```python
from build123d import *

# Parameters (mm, degrees)
F0_W     = 180
F0_H     = 270
F0_W_2   = 140
F0_H_2   = 230
F1_DEPTH = 11


with BuildPart() as f1:
    # F0 (on Right) → F1 (new body)
    with BuildSketch(Plane.YZ):
        with Locations((-34.164113, -2.262233)):
            Rectangle(F0_W, F0_H)
        with Locations((-34.164113, -2.262233)):
            Rectangle(F0_W_2, F0_H_2, mode=Mode.SUBTRACT)
    extrude(amount=F1_DEPTH)


solid = f1.part
```
Read the model definition and answer for the solid it produces. Units are mm, in the model's axes. A direction names the side the tool comes from. Give positions to 0.01 mm unless a question says otherwise; leave off trailing zeros. Order: outer loops, then holes, each group sorted by start corner. A loop starts at its lowest first (then second) coordinate and runs counter-clockwise, first axis right, second up.
(1) For a pull along Y with two mould halves and no side action, classify faces 3 (the flat face through (5, -124.164, -4)), 4 (the flat face through (5, -35, 132.738)), 5 (the flat face through (5, 35.836, -4)), 6 (the flat face through (5, 55.836, -4)) as released by +Y, released by -Y, zero draft, split by the parting line, or undercut.
(2) Find section C-C (x = 7.75). Give the vertices of the cut face in (y, z), plus the area to 3 significant figures.
(3) Find section B-B (z = -9). Give the vertices of the cut face in (x, y), plus the area to 3 significant figures.
(4) Find section A-A (y = 22). Give the vertices of the cut face in (x, z).
(5) Given pin 1 (10 mm diameter, centred on y = 26, z = 60, fed in from -X), flat-ended and moving along its own axis, determine where the tip first touches the part or whether it passes through.
(6) Straight lines are drawn through the part: L1, parallel to Z at x = 3.25, y = 35.5; L2, parallel to Y at x = 9.75, z = -43. For each, find the intervals that lie inside material, in ascending order.
(7) For faces 1 (the flat face through (5, -35, 112.738)), 2 (the flat face through (11, -115, 0)), determine the directions among +Z, -Z, +X, -X, +Y, -Y from which every point of the face is accessible in a straight line to the end or side of a thin tool.
Result sheet:
1. face 3: released by -Y
1. face 4: zero draft
1. face 5: undercut
1. face 6: released by +Y
2. outline: (-124.16, -137.26) - (55.84, -137.26) - (55.84, 132.74) - (-124.16, 132.74) - close; hole (-104.16, -117.26) - (35.84, -117.26) - (35.84, 112.74) - (-104.16, 112.74) - close
2. area: 16,400 mm2
3. outline: (0, -124.16) - (11, -124.16) - (11, -104.16) - (0, -104.16) - close; (0, 35.84) - (11, 35.84) - (11, 55.84) - (0, 55.84) - close
3. area: 440 mm2
4. outline: (0, -137.26) - (11, -137.26) - (11, -117.26) - (0, -117.26) - close; (0, 112.74) - (11, 112.74) - (11, 132.74) - (0, 132.74) - close
5. pin 1: passes through
6. L1: z = -137.26 to -117.26, 112.74 to 132.74
6. L2: y = -124.16 to -104.16, 35.84 to 55.84
7. face 1: +X, -X
7. face 2: +Z, -Z, +X, +Y, -Y
